Input: part model. Units: mm. Frame: model coordinates. A direction names the side the tool comes from. Coordinates: 2 decimals unless noted, no trailing zeros. Loops run counter-clockwise (first coordinate to the right, second up) from the corner with the lowest first, then second, coordinate; pieces in that order, holes last.
Item 1: Ray query, line 1 along X through (y, z) = (-10, 2); line 2 along Z through (x, y) = (-10, -11.7); line 3 along Z through (x, y) = (4.5, -2.25). Return the intervals inside material, ascending.
Item 2: Section A-A on z = 4. Return loops of the section in (x, y).
Item 3: Contact query for flat-ended pins moving along their axis: P1, Ø1.2, axis at y = 12.5, z = 3.5, coming from the -X side; P2, Ø1.4, axis at x = -10, z = 2.5, coming from the -Y side; P3, Ø6.5, axis at x = -6.5, y = 0, coming from the -Z side. Output: stop coordinate, or through.
Item 4: Reachability of faces 1 (the cylindrical face through (6.956, -1.309, -1.986)), 2 (the flat face through (0, 9.5, 2)), 3 (the cylindrical face through (10.77, -11.47, 2.26)) from +Z, -Z, +X, -X, +Y, -Y: full face, straight path, thin tool, end or side. Return the list, or none.
Item 5: Pull-direction query (Z, two-part tool) for faces 4 (the conical face through (-9.861, -9.103, 2.494)), 5 (the cylindrical face through (-16.93, -5.12, 4.4)), 6 (the flat face through (9, 1, -1)), 7 (the cylindrical face through (-7.068, -1.15, 2.042)); classes: released by +Z, released by -Z, zero draft, split by the parting line, or undercut.
Item 6: Section B-B on z = -2. Return loops of the section in (x, y), and give its area (3 significant figures).
```python
from build123d import *

# Parameters (mm, degrees)
BOSS_EXTRUDE1_DEPTH              = 5
FILLET1_R                        = 10
FILLET2_R                        = 2
SKETCH2_R                        = 6.5
SKETCH2_R_2                      = 2.3
SKETCH2_R_3                      = 6.2
BOSS_EXTRUDE2_DEPTH              = 1
FILLET3_R                        = 1.5
TAP_DRILL_SLOT_FOR_M2_TAP1_D     = 1.6
TAP_DRILL_SLOT_FOR_M2_TAP1_DEPTH = 4
TAP_DRILL_SLOT_FOR_M2_TAP1_TIP   = 0.480688495
SKETCH3_R                        = 2.3
BOSS_EXTRUDE3_DEPTH              = 2
SKETCH8_R                        = 2.3
CUT_EXTRUDE1_DEPTH               = 10


with BuildPart() as part:
    # Sketch1 → Boss-Extrude1 (new body)
    with BuildSketch(Plane.XY):
        Polygon((3, 13.5), (3, 9.5), (-3, 9.5), (-3, 13.5), (-17.5, 13.5), (-17.5, -13.5), (17.5, -13.5), (17.5, 13.5), align=None)
    extrude(amount=BOSS_EXTRUDE1_DEPTH)

    # Fillet1
    fillet1_edges = [part.edges().sort_by_distance(p)[0] for p in [
        (17.5, 13.5, 2.5),
        (-17.5, 13.5, 2.5),
    ]]
    fillet(fillet1_edges, radius=FILLET1_R)

    # Fillet2
    fillet2_edges = [part.edges().sort_by_distance(p)[0] for p in [
        (-5.25, 13.5, 5),
        (-17.5, -5, 5),
        (17.5, -5, 5),
        (5.25, 13.5, 5),
        (14.571067812, 10.571067812, 5),
        (-14.571067812, 10.571067812, 5),
    ]]
    fillet(fillet2_edges, radius=FILLET2_R)

    # Sketch2 → Boss-Extrude2 (add)
    # profile 1 of 2: a face of its own
    with BuildSketch(Plane(origin=(0, 0, 0), x_dir=(-1, 0, 0), z_dir=(0, 0, -1))):
        with Locations(Location((9.261392854, -1.840391381, 0), (0, 0, 180))):
            Circle(SKETCH2_R)
        with Locations((9.261392854, -1.840391381)):
            Circle(SKETCH2_R_2, mode=Mode.SUBTRACT)
    # profile 2 of 2: a face of its own
    with BuildSketch(Plane(origin=(0, 0, 0), x_dir=(-1, 0, 0), z_dir=(0, 0, -1))):
        with Locations(Location((-9.15, -2, 0), (0, 0, 180))):
            Circle(SKETCH2_R_3)
    extrude(amount=BOSS_EXTRUDE2_DEPTH)

    # Fillet3
    # the kernel refuses this fillet: 1.5 mm, written as the material it adds along each edge
    with BuildSketch(Plane(origin=(-9.261392854, -1.840391381, 0), x_dir=(1, 0, 0), z_dir=(0, 1, 0))) as fillet3_piece_1:
        with BuildLine():
            CenterArc((7.914213562, 1.5), FILLET3_R, 199.471220634, 70.528779366)
            Line((6.5, 1), (6.471715729, 0.99))
            ThreePointArc((6.471715729, 0.99), (6.47, 0.5), (6.47, 0))
            Line((6.47, 0), (6.5, -0.03))
            Line((6.5, -0.03), (7.914213562, -0.03))
            Line((7.914213562, -0.03), (7.914213562, 0))
        make_face()
    revolve(axis=Axis((-9.261392854, -1.840391381, 0), (0, 0, -1)))
    with BuildSketch(Plane(origin=(9.15, -2, 0), x_dir=(1, 0, 0), z_dir=(0, 1, 0))) as fillet3_piece_2:
        with BuildLine():
            CenterArc((7.614213562, 1.5), FILLET3_R, 199.471220634, 70.528779366)
            Line((6.2, 1), (6.171715729, 0.99))
            ThreePointArc((6.171715729, 0.99), (6.17, 0.5), (6.17, 0))
            Line((6.17, 0), (6.2, -0.03))
            Line((6.2, -0.03), (7.614213562, -0.03))
            Line((7.614213562, -0.03), (7.614213562, 0))
        make_face()
    revolve(axis=Axis((9.15, -2, 0), (0, 0, -1)))

    # Tap Drill Slot for M2 Tap1
    with Locations(Plane(origin=(0, -13.5, 0), x_dir=(-1, 0, 0), z_dir=(0, -1, 0))):
        with Locations((-10.007456689, -2.505236507), (0, -2.505236507), (10, -2.5)):
            Hole(TAP_DRILL_SLOT_FOR_M2_TAP1_D / 2, depth=TAP_DRILL_SLOT_FOR_M2_TAP1_DEPTH)
            with Locations((0, 0, -(TAP_DRILL_SLOT_FOR_M2_TAP1_DEPTH + TAP_DRILL_SLOT_FOR_M2_TAP1_TIP / 2))):  # 118° drill point
                Cone(0, TAP_DRILL_SLOT_FOR_M2_TAP1_D / 2, TAP_DRILL_SLOT_FOR_M2_TAP1_TIP, mode=Mode.SUBTRACT)

    # Sketch3 → Boss-Extrude3 (add)
    with BuildSketch(Plane(origin=(0, 0, -1), x_dir=(-1, 0, 0), z_dir=(0, 0, -1))):
        with Locations((-9.15, -2)):
            Circle(SKETCH3_R)
    extrude(amount=BOSS_EXTRUDE3_DEPTH)

    # Sketch8 → Cut-Extrude1 (cut)
    with BuildSketch(Plane.XY.offset(5)):
        with Locations((-9.261392854, -1.840391381)):
            Circle(SKETCH8_R)
    extrude(amount=-CUT_EXTRUDE1_DEPTH, mode=Mode.SUBTRACT)


solid = part.part
```
Results found:
1. line 1: x = -17.5 to -10.62, -9.38 to -0.62, 0.62 to 9.39, 10.63 to 17.5
1. line 2: z = 0 to 1.7, 3.3 to 5
1. line 3: z = -1 to 5
2. outline: (-17.23, -13.5) - (17.23, -13.5) - (17.23, 3.5) arc R9.73 ccw to (7.5, 13.23) - (3, 13.23) - (3, 9.5) - (-3, 9.5) - (-3, 13.23) - (-7.5, 13.23) arc R9.73 ccw to (-17.23, 3.5) - close; hole circle Ø4.6 at (-9.26, -1.84)
3. P1: stops at x = -12.84
3. P2: stops at y = -9.44
3. P3: stops at z = -1
4. face 1: -Z
4. face 2: +Z, -Z, +Y
4. face 3: -Y
5. face 4: undercut
5. face 5: released by +Z
5. face 6: released by -Z
5. face 7: zero draft
6. outline: circle Ø4.6 at (9.15, -2)
6. area: 16.6 mm2
